from build123d import *

# Parameters (mm, degrees)
F1_DEPTH = 19.05


with BuildPart() as f1:
    # F0 (on Top) → F1 (new body)
    with BuildSketch(Plane.XY):
        Polygon((0, -152.4), (0, 0), (-38.1, 0), (-38.1, -63.5), (-38.1, -88.9), (-38.1, -152.4), align=None)
        Polygon((-38.1, -63.5), (-38.1, 0), (-292.1, 0), (-292.1, -63.5), (-273.05, -63.5), (-273.05, -88.9), (-292.1, -88.9), (-292.1, -152.4), (-38.1, -152.4), (-38.1, -88.9), (-57.15, -88.9), (-57.15, -63.5), align=None)
        Polygon((-292.1, -63.5), (-292.1, 0), (-330.2, 0), (-330.2, -152.4), (-292.1, -152.4), (-292.1, -88.9), align=None)
    extrude(amount=F1_DEPTH)


solid = f1.part
Input: part model. Units: mm. Frame: model coordinates. A direction names the side the tool comes from. Coordinates: 2 decimals unless noted, no trailing zeros. Order: outer loops, then holes, each group sorted by start corner. A loop starts at its lowest first (then second) coordinate and runs counter-clockwise, first axis right, second up. Notation, with made-up numbers: M 30,-7.75 L 47,-7.75 A24 cw 47,23.25 Z; hole C 20.5,71 d8. An arc over 180 degrees is marked long. Answer as CSV lines item,"result".
1. Pull-direction query (Y, two-part tool) for faces 1 (the flat face through (-167, -152.4, 9)), 2 (the flat face through (-273.05, -76, 9)), 3 (the flat face through (-330.2, -75, 9)); classes: released by +Y, released by -Y, zero draft, split by the parting line, or undercut.
Reported:
face 1,"released by -Y"
face 2,"undercut"
face 3,"zero draft"
2. Access query for faces 4 (the flat face through (-283, -63.5, 9)), 5 (the flat face through (-163, 0, 9)). Directions: +Z, -Z, +X, -X, +Y, -Y. A direction counts if a zero-diameter tool reaches every point of the face in a straight line with its end or side. Return the directions, or none.
Reported:
face 4,"+Z, -Z"
face 5,"+Z, -Z, +X, -X, +Y"
3. Section C-C (z = 10). Return the cut outline in (x, y), then the cut area to 3 significant figures.
Reported:
outline,"M -330.2,-152.4 L 0,-152.4 L 0,0 L -330.2,0 Z; hole M -292.1,-88.9 L -273.05,-88.9 L -273.05,-63.5 L -292.1,-63.5 Z; hole M -57.15,-88.9 L -38.1,-88.9 L -38.1,-63.5 L -57.15,-63.5 Z"
area,"49,400 mm2"
4. First-contact query: P1, Ø10, axis at x = -273.5, z = 7, coming from the +Y side. Flat tip, straight axial feed; report the tip coordinate or a pass-through.
Reported:
P1,"y = 0"
5. Section B-B (x = -285). Return the cut outline in (y, z), then the cut area to 3 significant figures.
Reported:
outline,"M -152.4,0 L -88.9,0 L -88.9,19.05 L -152.4,19.05 Z; M -63.5,0 L 0,0 L 0,19.05 L -63.5,19.05 Z"
area,"2,420 mm2"
6. Section A-A (y = -76.5). Return the cut outline in (x, z), then the cut area to 3 significant figures.
Reported:
outline,"M -330.2,0 L -292.1,0 L -292.1,19.05 L -330.2,19.05 Z; M -273.05,0 L -57.15,0 L -57.15,19.05 L -273.05,19.05 Z; M -38.1,0 L 0,0 L 0,19.05 L -38.1,19.05 Z"
area,"5,560 mm2"
7. Material intervals for line 1 (X direction, y = -79.5, z = 3.25); line 2 (Y direction, x = -290, z = 16.5), sorted ascending. Write a range as from..to.
Reported:
line 1,"-330.2..-292.1, -273.05..-57.15, -38.1..0"
line 2,"-152.4..-88.9, -63.5..0"
